Part model, mm, in its own coordinate system. A direction names the side the tool comes from. Round coordinates to 2 decimals unless told otherwise and drop trailing zeros. Loops run counter-clockwise (first coordinate to the right, second up) from the corner with the lowest first, then second, coordinate; pieces in that order, holes last.
1) Drop flat-ended pins along their axis: P1, Ø2, axis at x = -10.5, z = 6.5, coming from the +Y side; P2, Ø13.5, axis at x = -19, y = -22.5, coming from the +Z side; P3, Ø6, axis at x = -3.5, z = 6.5, coming from the -Y side; P4, Ø3.5, axis at x = -2, y = -58, coming from the -Z side. Give the stop position or say it passes through.
2) Band-saw the part on C-C, the plane z = -1. Write the cut outline in (x, y).
3) Probe line 1 (Z direction, x = -13, y = -4.25); line 2 (Z direction, x = -13, y = -2.75); line 3 (X direction, y = -58, z = 0.1). List the from-to ranges inside material, lowest first.
4) Mould opens along Z. For faces 1 (the flat face through (-2, -59, 4.75)), 2 (the flat face through (-15, -2, -2.5)), 3 (the flat face through (-27, -3, 2)) say: +Z half, -Z half, draft (parallel to the pull), parting line (faces both ways), or undercut.
5) Band-saw the part on B-B, the plane x = -13. Write the cut outline in (y, z), then the cut area to 3 significant figures.
6) Band-saw the part on A-A, the plane x = -6.5. Write the cut outline in (y, z).
7) 3-axis set-ups, long thin cutter, end or side, ignore diameter. For faces 4 (the flat face through (-15, -4, -1)), 5 (the flat face through (-15, -4, 6)), 6 (the flat face through (-15, -1, 6)), 7 (the flat face through (-1, -53, 3)): which of +Z, -Z, +X, -X, +Y, -Y reach the whole face in a straight line?
8) Band-saw the part on D-D, the plane y = -11. Write the cut outline in (x, z).
from build123d import *

# Parameters (mm, degrees)
BOSS_EXTRUDE1_DEPTH = 5
FILLET1_R           = 3
SKETCH2_W           = 24
SKETCH2_H           = 3
BOSS_EXTRUDE2_DEPTH = 2.5
SKETCH3_W           = 24
SKETCH3_H           = 3
BOSS_EXTRUDE3_DEPTH = 2.5
SKETCH4_W           = 5
SKETCH4_H           = 6.1
CUT_EXTRUDE1_DEPTH  = 1
SKETCH5_R           = 1.5
CUT_EXTRUDE2_DEPTH  = 14
SKETCH7_R           = 0.25
CUT_EXTRUDE3_DEPTH  = 10
SKETCH8_W           = 4.5
SKETCH8_H           = 3
CUT_EXTRUDE4_DEPTH  = 5
SKETCH12_R          = 0.5
BOSS_EXTRUDE4_DEPTH = 0.5
SKETCH13_R          = 0.4
CUT_EXTRUDE5_DEPTH  = 3.5


with BuildPart() as part:
    # Sketch1 → Boss-Extrude1 (new body)
    with BuildSketch(Plane.XY):
        with BuildLine():
            Line((0, -60), (-5, -60))
            Line((-5, -60), (-5, -40))
            Line((-5, -40), (-12, -5))
            Line((-12, -5), (-27, -5))
            Line((-27, -5), (-27, 0))
            Line((-27, 0), (-3, 0))
            Line((-3, 0), (-3, -27.2))
            ThreePointArc((-3, -27.2), (-2.179898987, -29.179898987), (-0.2, -30))
            Line((-0.2, -30), (0, -30))
            Line((0, -30), (0, -60))
        make_face()
    extrude(amount=BOSS_EXTRUDE1_DEPTH)

    # Fillet1
    fillet1_edges = [part.edges().sort_by_distance(p)[0] for p in [
        (-5, -40, 2.5),
        (-12, -5, 2.5),
    ]]
    fillet(fillet1_edges, radius=FILLET1_R)

    # Sketch2 → Boss-Extrude2 (add)
    with BuildSketch(Plane.XY.offset(5)):
        with Locations((-15, -2.5)):
            Rectangle(SKETCH2_W, SKETCH2_H)
    extrude(amount=BOSS_EXTRUDE2_DEPTH)

    # Sketch3 → Boss-Extrude3 (add)
    with BuildSketch(Plane(origin=(0, 0, 0), x_dir=(-1, 0, 0), z_dir=(0, 0, -1))):
        with Locations((15, -2.5)):
            Rectangle(SKETCH3_W, SKETCH3_H)
    extrude(amount=BOSS_EXTRUDE3_DEPTH)

    # Sketch4 → Cut-Extrude1 (cut)
    with BuildSketch(Plane(origin=(0, 0, 0), x_dir=(0, 0, -1), z_dir=(1, 0, 0))):
        with Locations((-2.5, -52.95)):
            Rectangle(SKETCH4_W, SKETCH4_H)
        with Locations((-2.5, -42.85)):
            Rectangle(SKETCH4_W, SKETCH4_H)
        with Locations((-2.5, -32.75)):
            Rectangle(SKETCH4_W, SKETCH4_H)
        with Locations((-2.5, -22.65)):
            Rectangle(SKETCH4_W, SKETCH4_H)
        with Locations((-2.5, -12.55)):
            Rectangle(SKETCH4_W, SKETCH4_H)
        with Locations((-2.5, -2.45)):
            Rectangle(SKETCH4_W, SKETCH4_H)
    extrude(amount=-CUT_EXTRUDE1_DEPTH, mode=Mode.SUBTRACT)

    # Sketch5 → Cut-Extrude2 (cut)
    with BuildSketch(Plane(origin=(0, 0, 0), x_dir=(1, 0, 0), z_dir=(0, 1, 0))):
        with Locations(Location((-13, -2.5, 0), (0, 0, 180))):
            Circle(SKETCH5_R)
    extrude(amount=-CUT_EXTRUDE2_DEPTH, mode=Mode.SUBTRACT)

    # Sketch7 → Cut-Extrude3 (cut)
    with BuildSketch(Plane.XY.offset(5)):
        with Locations((-2.5, -58)):
            Circle(SKETCH7_R)
    extrude(amount=-CUT_EXTRUDE3_DEPTH, mode=Mode.SUBTRACT)

    # Sketch8 → Cut-Extrude4 (cut)
    with BuildSketch(Plane(origin=(0, 0, 0), x_dir=(0, 0, -1), z_dir=(1, 0, 0))):
        with Locations((-2.5, -58.5)):
            Rectangle(SKETCH8_W, SKETCH8_H)
    extrude(amount=-CUT_EXTRUDE4_DEPTH, mode=Mode.SUBTRACT)

    # Sketch12 → Boss-Extrude4 (add)
    with BuildSketch(Plane(origin=(0, 0, 0), x_dir=(0, 0, -1), z_dir=(1, 0, 0))):
        with Locations(Location((-2.5, -47.9, 0), (0, 0, 270))):
            Circle(SKETCH12_R)
    extrude(amount=BOSS_EXTRUDE4_DEPTH)

    # Sketch13 → Cut-Extrude5 (cut)
    with BuildSketch(Plane(origin=(0.5, 0, 0), x_dir=(0, 0, -1), z_dir=(1, 0, 0))):
        with Locations(Location((-2.5, -47.9, 0), (0, 0, 90))):
            Circle(SKETCH13_R)
    extrude(amount=-CUT_EXTRUDE5_DEPTH, mode=Mode.SUBTRACT)


solid = part.part
Reported:
1. P1: stops at y = -1
1. P2: passes through
1. P3: stops at y = -60
1. P4: stops at z = 0
2. outline: (-27, -4) - (-3, -4) - (-3, -1) - (-27, -1) - close
3. line 1: z = 0 to 1, 4 to 5
3. line 2: z = -2.5 to 1, 4 to 7.5
3. line 3: x = -5 to -2.75, -2.25 to 0
4. face 1: undercut
4. face 2: -Z half
4. face 3: draft
5. outline: (-5.38, 0) - (-4, 0) - (-4, -2.5) - (-1, -2.5) - (-1, 0) - (0, 0) - (0, 1) - (-5.38, 1) - close; (-5.38, 4) - (0, 4) - (0, 5) - (-1, 5) - (-1, 7.5) - (-4, 7.5) - (-4, 5) - (-5.38, 5) - close
5. area: 25.8 mm2
6. outline: (-32.5, 0) - (-4, 0) - (-4, -2.5) - (-1, -2.5) - (-1, 0) - (0, 0) - (0, 5) - (-1, 5) - (-1, 7.5) - (-4, 7.5) - (-4, 5) - (-32.5, 5) - close
7. face 4: -Z, +X, -X, -Y
7. face 5: +Z, +X, -X, -Y
7. face 6: +Z, +X, -X, +Y
7. face 7: +Z, -Z, +X
8. outline: (-10.8, 0) - (-3, 0) - (-3, 5) - (-10.8, 5) - close
